Geometry check sheet. Reference: the model listing, model coordinates, mm. Face numbers are marked on the shaded views. A direction names the side the tool comes from. Coordinates: 2 decimals unless noted, no trailing zeros. Write each loop counter-clockwise with the first axis right and the second up, starting at its lowest first coordinate (ties: lowest second). Pieces come first, ordered by that corner, then holes.
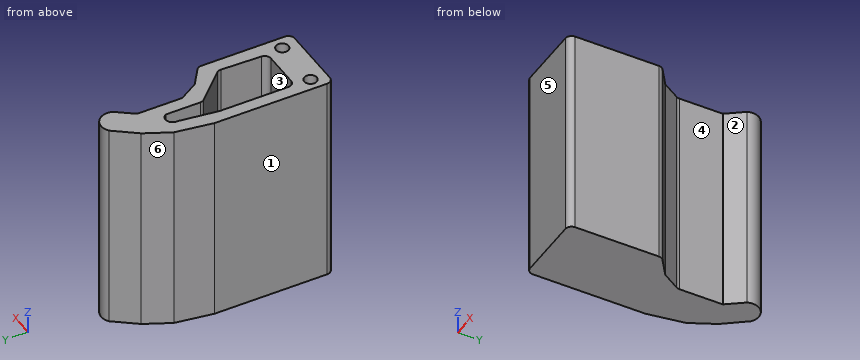
from build123d import *

# Parameters (mm, degrees)
BOSS_EXTRUDE1_DEPTH = 34
CUT_EXTRUDE1_DEPTH  = 32
SKETCH3_R           = 1
CUT_EXTRUDE2_DEPTH  = 32
FILLET2_R           = 1


with BuildPart() as part:
    # Sketch1 → Boss-Extrude1 (new body)
    with BuildSketch(Plane.XY.offset(40)):
        with BuildLine():
            Line((-300, 367), (-300, 348))
            Line((-300, 348), (-287.95160644, 348))
            Line((-287.95160644, 348), (-287.95160644, 362.871836257))
            Line((-287.95160644, 362.871836257), (-291.110931396, 365.166412354))
            Line((-291.110931396, 365.166412354), (-292.925810618, 368.159105691))
            Line((-292.925810618, 368.159105691), (-292.925810618, 375.359105691))
            Line((-292.925810618, 375.359105691), (-290.910509572, 378.097455869))
            ThreePointArc((-290.910509572, 378.097455869), (-291.625724396, 380.675408146), (-294.299987793, 380.600006104))
            Line((-294.299987793, 380.600006104), (-297.012375964, 377.009330623))
            Line((-297.012375964, 377.009330623), (-299.029605392, 372.921007879))
            Line((-299.029605392, 372.921007879), (-300, 367))
        make_face()
    extrude(amount=BOSS_EXTRUDE1_DEPTH)

    # Sketch2 → Cut-Extrude1 (cut)
    with BuildSketch(Plane.XY.offset(74)):
        with BuildLine():
            Line((-297.116612998, 371.207677878), (-298, 365))
            Line((-298, 365), (-298, 353.070416706))
            Line((-298, 353.070416706), (-290.26344591, 353.070416706))
            Line((-290.26344591, 353.070416706), (-290.018829346, 360.778991699))
            Line((-290.018829346, 360.778991699), (-295.010009766, 366.046598155))
            Line((-295.010009766, 366.046598155), (-295.010009766, 371.995180703))
            ThreePointArc((-295.010009766, 371.995180703), (-296.391652801, 372.479756418), (-297.116612998, 371.207677878))
        make_face()
    extrude(amount=-CUT_EXTRUDE1_DEPTH, mode=Mode.SUBTRACT)

    # Sketch3 → Cut-Extrude2 (cut)
    with BuildSketch(Plane.XY.offset(74)):
        with Locations((-298.046417962, 350.546056216)):
            Circle(SKETCH3_R)
        with Locations((-289.979523898, 350.546056216)):
            Circle(SKETCH3_R)
    extrude(amount=-CUT_EXTRUDE2_DEPTH, mode=Mode.SUBTRACT)

    # Fillet2
    fillet2_edges = [part.edges().sort_by_distance(p)[0] for p in [
        (-292.925810618, 368.159105691, 57),
        (-287.95160644, 362.871836257, 57),
        (-287.95160644, 348, 57),
        (-300, 348, 57),
        (-295.010009766, 366.046598155, 58),
        (-290.018829346, 360.778991699, 58),
        (-290.26344591, 353.070416706, 58),
        (-298, 353.070416706, 58),
    ]]
    fillet(fillet2_edges, radius=FILLET2_R)


solid = part.part
1. Thickness scan on line 1 along X through (y, z) = (354, 57); line 2 along X through (y, z) = (367, 69); line 3 along Y through (x, z) = (-294.75, 70.5). Record the ranges inside material, lowest first.
Computed values:
line 1: x = -300 to -298, -290.23 to -287.95
line 2: x = -300 to -297.72, -295.01 to -292.22
line 3: y = 348 to 353.07, 365.77 to 380
2. Sectioned sample at A-A, the plane z = 49.5. Record the boundary of the cut face in (x, y).
Computed values:
outline: (-300, 349) arc R1 ccw to (-299, 348) - (-288.95, 348) arc R1 ccw to (-287.95, 349) - (-287.95, 362.36) arc R1 ccw to (-288.36, 363.17) - (-291.11, 365.17) - (-292.78, 367.92) arc R1 cw to (-292.93, 368.44) - (-292.93, 375.36) - (-290.91, 378.1) arc R2.17 ccw to (-294.3, 380.6) - (-297.01, 377.01) - (-299.03, 372.92) - (-300, 367) - close; hole circle Ø2 at (-298.05, 350.55); hole (-298, 354.07) arc R1 ccw to (-297, 353.07) - (-291.23, 353.07) arc R1 ccw to (-290.23, 354.04) - (-290.03, 360.36) arc R1 ccw to (-290.31, 361.08) - (-294.74, 365.76) arc R1 cw to (-295.01, 366.45) - (-295.01, 372) arc R1.14 ccw to (-297.12, 371.21) - (-298, 365) - close; hole circle Ø2 at (-289.98, 350.55)
3. Sectioned sample at D-D, the plane x = -299.5. Record the boundary of the cut face in (y, z).
Computed values:
outline: (348.13, 40) - (370.05, 40) - (370.05, 74) - (348.13, 74) - close
4. Draft check along Y on the marked faces 3, 4, 5 and 6. Enter one of: released by +Y, released by -Y, zero draft, split by the parting line, or undercut.
Computed values:
face 3: undercut
face 4: undercut
face 5: released by -Y
face 6: released by +Y
5. Sectioned sample at C-C, the plane x = -296.5. Record the boundary of the cut face in (y, z).
Computed values:
outline: (348, 40) - (377.69, 40) - (377.69, 74) - (372.43, 74) - (372.43, 42) - (353.07, 42) - (353.07, 74) - (348, 74) - close
6. Access from +Z, -Z, +X, -X, +Y, -Y to the whole of each face (thin tool, end or side, straight path). Record for the marked faces 1 and 2.
Computed values:
face 1: +Z, -Z, -X, +Y, -Y
face 2: +Z, -Z, +X
7. Sectioned sample at B-B, the plane y = 370. Record the boundary of the cut face in (x, z), and give its area (3 significant figures).
Computed values:
outline: (-299.51, 40) - (-292.93, 40) - (-292.93, 74) - (-295.01, 74) - (-295.01, 42) - (-297.29, 42) - (-297.29, 74) - (-299.51, 74) - close
area: 151 mm2
8. Gauge pin test, flat ends, axial feed: pin 1 Ø1.5 at (y, z) = (367, 63.5) entering from +X; pin 2 Ø3 at (x, y) = (-298.05, 350.55) entering from +Z; pin 3 Ø0.6 at (x, y) = (-290, 350.5) entering from +Z; pin 4 Ø1.5 at (x, z) = (-295.5, 63.5) entering from +Y. Record the tip position at first contact, or that the pin passes through.
Computed values:
pin 1: stops at x = -291.77
pin 2: stops at z = 74
pin 3: stops at z = 42
pin 4: stops at y = 380
